The listing builds one solid part. Answer for the finished solid, in the listing's coordinates (mm). Coordinates: 2 decimals unless noted, no trailing zeros. Order: outer loops, then holes, each group sorted by start corner. A loop starts at its lowest first (then second) coordinate and runs counter-clockwise, first axis right, second up. Notation, with made-up numbers: (62.25, 84.5) - (79.25, 84.5) arc R25 ccw to (79.25, 97.5) - close; hole circle Ø10 at (19, 40.25). An arc over 180 degrees is marked (long way). Use a Markdown table: item, result. Add a question column.
Item 1: Flat-ended cylindrical pins translate along their axes: P1, Ø1.5, axis at x = 1, y = 8, coming from the +Z side; P2, Ø3.5, axis at y = -6.01, z = 6.01, coming from the +X side; P3, Ø1, axis at x = 0.5, z = -1.5, coming from the -Y side. Find the tip coordinate at first contact, or state that the pin passes through.
Item 2: The part is cut by section C-C, the plane x = 0.3. Give the vertices of the cut face in (y, z), then the cut area to 3 significant figures.
Item 3: The mould has two halves that part along Y. Classify faces 1 (the cylindrical face through (1.479, 4.461, 4.864)), 2 (the cylindrical face through (1.48, -10.74, 2.38)), 3 (the flat face through (0, -5, -5)): released by +Y, released by -Y, zero draft, split by the parting line, or undercut.
Item 4: The part is cut by section A-A, the plane z = 0. Give the vertices of the cut face in (x, y), then the cut area to 3 significant figures.
Item 5: Find the intervals of material crossed by line 1 along Y through (x, z) = (0.5, -0.25); line 2 along Y through (x, z) = (1.8, -6); line 3 along Y through (x, z) = (1.7, 1.25), in increasing order.
Item 6: The part is cut by section D-D, the plane z = -9.5. Give the vertices of the cut face in (x, y).
from build123d import *

# Parameters (mm, degrees)
SKETCH2_R           = 11
SKETCH2_R_2         = 6.6
BOSS_EXTRUDE1_DEPTH = 3
SKETCH3_R           = 1.15
CUT_EXTRUDE1_DEPTH  = 4


with BuildPart() as part:
    # Sketch2 → Boss-Extrude1 (new body)
    with BuildSketch(Plane(origin=(0, 0, 0), x_dir=(0, 0, -1), z_dir=(1, 0, 0))):
        Circle(SKETCH2_R)
        Circle(SKETCH2_R_2, mode=Mode.SUBTRACT)
    extrude(amount=BOSS_EXTRUDE1_DEPTH)

    # Sketch3 → Cut-Extrude1 (cut, through all)
    with BuildSketch(Plane(origin=(0, 0, 0), x_dir=(0, 0, -1), z_dir=(1, 0, 0))):
        with Locations((6.01040764, 6.01040764)):
            Circle(SKETCH3_R)
        with Locations((6.01040764, -6.01040764)):
            Circle(SKETCH3_R)
        with Locations((-6.01040764, -6.01040764)):
            Circle(SKETCH3_R)
        with Locations((-6.01040764, 6.01040764)):
            Circle(SKETCH3_R)
    extrude(amount=CUT_EXTRUDE1_DEPTH, mode=Mode.SUBTRACT)


solid = part.part
Solution:
| question | item | result |
|---|---|---|
| 1 | P1 | stops at z = 8.27 |
| 1 | P2 | stops at x = 3 |
| 1 | P3 | stops at y = -10.95 |
| 2 | outline | circle Ø22 at (0, 0); hole circle Ø2.3 at (-6.01, -6.01); hole circle Ø2.3 at (-6.01, 6.01); hole circle Ø13.2 at (0, 0); hole circle Ø2.3 at (6.01, -6.01); hole circle Ø2.3 at (6.01, 6.01) |
| 2 | area | 227 mm2 |
| 3 | face 1 | undercut |
| 3 | face 2 | split by the parting line |
| 3 | face 3 | zero draft |
| 4 | outline | (0, -11) - (3, -11) - (3, -6.6) - (0, -6.6) - close; (0, 6.6) - (3, 6.6) - (3, 11) - (0, 11) - close |
| 4 | area | 26.4 mm2 |
| 5 | line 1 | y = -11 to -6.6, 6.6 to 11 |
| 5 | line 2 | y = -9.22 to -7.16, -4.86 to -2.75, 2.75 to 4.86, 7.16 to 9.22 |
| 5 | line 3 | y = -10.93 to -6.48, 6.48 to 10.93 |
| 6 | outline | (0, -5.55) - (3, -5.55) - (3, 5.55) - (0, 5.55) - close |
